Check sheet for the modelled part. Datum: model origin and axes. Units: mm. A direction names the side the tool comes from. Round coordinates to 2 decimals unless told otherwise and drop trailing zeros. Write each loop counter-clockwise with the first axis right and the second up, starting at its lowest first coordinate (ties: lowest second). Pieces come first, ordered by that corner, then holes.
Item 1: Tool access check on faces 5 (the flat face through (44, 37, 20)), 6 (the flat face through (24, 0, 37)). Record the directions out of +Z, -Z, +X, -X, +Y, -Y that give a thin tool (end or side, any length) a straight path to the whole face; none if there is none.
Item 2: Release check for a two-part mould opening along Z. For faces 1 (the flat face through (31, 38, 0)), 2 (the flat face through (25, 37, 38)), 3 (the flat face through (63, 37, 65)), 4 (the flat face through (44, 38, 55)) record: +Z half, -Z half, draft (parallel to the pull), parting line (faces both ways), or undercut.
Item 3: Go/stop test with a flat-tipped pin: pin 1 Ø10.5 at (y, z) = (41, 37) entering from +X. Record where the tip stops, or that it passes through.
Item 4: Cross-section at A-A on x = 32. Enter the section's corners in (y, z), plus the area to 3 significant figures.
Item 5: Cross-section at B-B on y = 48. Enter the section's corners in (x, z), plus the area to 4 significant figures.
Item 6: Material ranges on line 1 (Z direction, x = 42, y = 67); line 2 (X direction, y = 23, z = 53), recorded low to high.
Item 7: Cross-section at C-C on z = 24.5. Enter the section's corners in (x, y).
from build123d import *

# Parameters (mm, degrees)
F0_W     = 63
F0_H     = 75
F1_DEPTH = 75
F3_DEPTH = 38


with BuildPart() as f1:
    # F0 (on Top) → F1 (new body)
    with BuildSketch(Plane.XY):
        with Locations((31.5, 37.5)):
            Rectangle(F0_W, F0_H)
    extrude(amount=F1_DEPTH)

    # F2 (on face) → F3 (cut)
    with BuildSketch(Plane.YZ.offset(63)):
        Polygon((0, 20), (37.5, 20), (75, 20), (75, 55), (0, 55), align=None)
    extrude(amount=-F3_DEPTH, mode=Mode.SUBTRACT)


solid = f1.part
Response values:
1. face 5: +X, +Y, -Y
1. face 6: +Z, -Z, +X, -X, -Y
2. face 1: -Z half
2. face 2: undercut
2. face 3: draft
2. face 4: undercut
3. pin 1: stops at x = 25
4. outline: (0, 0) - (75, 0) - (75, 20) - (0, 20) - close; (0, 55) - (75, 55) - (75, 75) - (0, 75) - close
4. area: 3,000 mm2
5. outline: (0, 0) - (63, 0) - (63, 20) - (25, 20) - (25, 55) - (63, 55) - (63, 75) - (0, 75) - close
5. area: 3,395 mm2
6. line 1: z = 0 to 20, 55 to 75
6. line 2: x = 0 to 25
7. outline: (0, 0) - (25, 0) - (25, 75) - (0, 75) - close
